Job drawing, mm, ordinate dimensions from the low corner. One solid piece. A direction names the side the tool comes from. Coordinates: 2 decimals unless noted, no trailing zeros. Write each loop counter-clockwise with the first axis right and the second up, starting at its lowest first coordinate (ties: lowest second). Pieces come first, ordered by that corner, then holes. Notation, with made-up numbers: M -18,20.5 L 24,20.5 A22 ccw 24,29.5 Z; hole C 38.25,58 d6. An arc over 180 degrees is marked long. Answer as CSV lines item,"result". Start each with the question number.
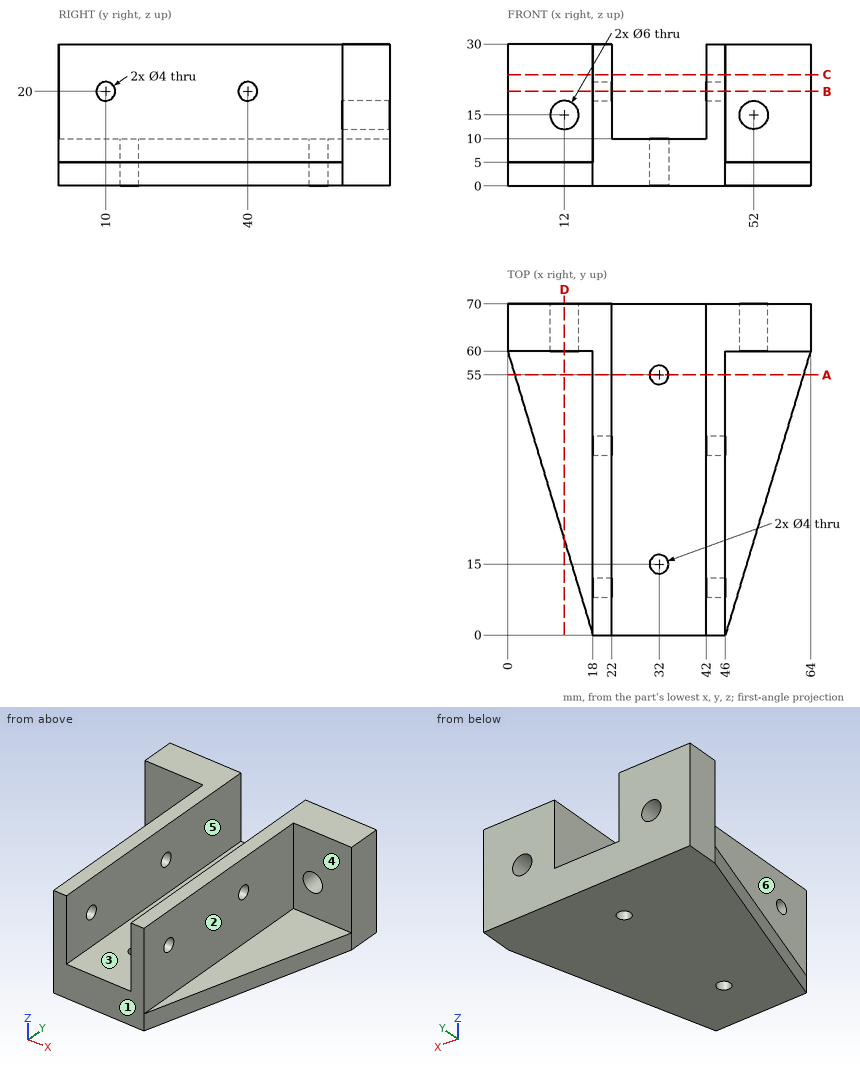
1) Band-saw the part on D-D, the plane x = 12. List the corners of the cut face in (y, z).
2) Pin check, flat tips, straight feed: P1, Ø1.5, axis at y = 15, z = 16.5, coming from the -X side; P2, Ø9, axis at x = 8.5, z = 22.5, coming from the -Y side; P3, Ø2.5, axis at y = 10, z = 20, coming from the +X side; P4, Ø5.5, axis at x = 12, y = 32.5, coming from the +Z side. Stop position of each tip, or through.
3) Band-saw the part on C-C, the plane z = 23.5. List the corners of the cut face in (x, y), plus the area to 3 significant figures.
4) Band-saw the part on B-B, the plane z = 20. List the corners of the cut face in (x, y).
5) Probe L1, parallel to X at y = 64.5, z = 15; L2, parallel to X at y = 31, z = 15.5; L3, parallel to Z at x = 19.2, y = 10. List the from-to ranges inside material, lowest first. Write a range as [from, to].
6) Band-saw the part on A-A, the plane y = 55. List the corners of the cut face in (x, z).
7) Two-plate mould, pull along X, no slides. Class the marked faces 1, 2 and 3: pulls with the +X half, pulls with the -X half, needs draft (parallel to the pull), parting line crosses it, or undercut.
8) Tool access for the marked faces 4, 5 and 6: list every direction of +Z, -Z, +X, -X, +Y, -Y with a clear straight run to the whole face (end or side of a thin tool).
Result sheet:
1,outline,"M 20,0 L 70,0 L 70,12 L 60,12 L 60,5 L 20,5 Z; M 60,18 L 70,18 L 70,30 L 60,30 Z"
2,P1,"stops at x = 18"
2,P2,"stops at y = 60"
2,P3,"passes through"
2,P4,"stops at z = 5"
3,outline,"M 0,60 L 18,60 L 18,0 L 22,0 L 22,70 L 0,70 Z; M 42,0 L 46,0 L 46,60 L 64,60 L 64,70 L 42,70 Z"
3,area,"920 mm²"
4,outline,"M 0,60 L 18,60 L 18,42 L 22,42 L 22,70 L 0,70 Z; M 18,0 L 22,0 L 22,8 L 18,8 Z; M 18,12 L 22,12 L 22,38 L 18,38 Z; M 42,0 L 46,0 L 46,8 L 42,8 Z; M 42,12 L 46,12 L 46,38 L 42,38 Z; M 42,42 L 46,42 L 46,60 L 64,60 L 64,70 L 42,70 Z"
5,L1,"x = [0, 9], [15, 22], [42, 49], [55, 64]"
5,L2,"x = [18, 22], [42, 46]"
5,L3,"z = [0, 18], [22, 30]"
6,outline,"M 1.5,0 L 30,0 L 30,10 L 22,10 L 22,30 L 18,30 L 18,5 L 1.5,5 Z; M 34,0 L 62.5,0 L 62.5,5 L 46,5 L 46,30 L 42,30 L 42,10 L 34,10 Z"
7,face 1,"needs draft"
7,face 2,"pulls with the +X half"
7,face 3,"undercut"
8,face 4,"+Z, +X, -Y"
8,face 5,"+Z, +Y, -Y"
8,face 6,"+Z, -X, -Y"
